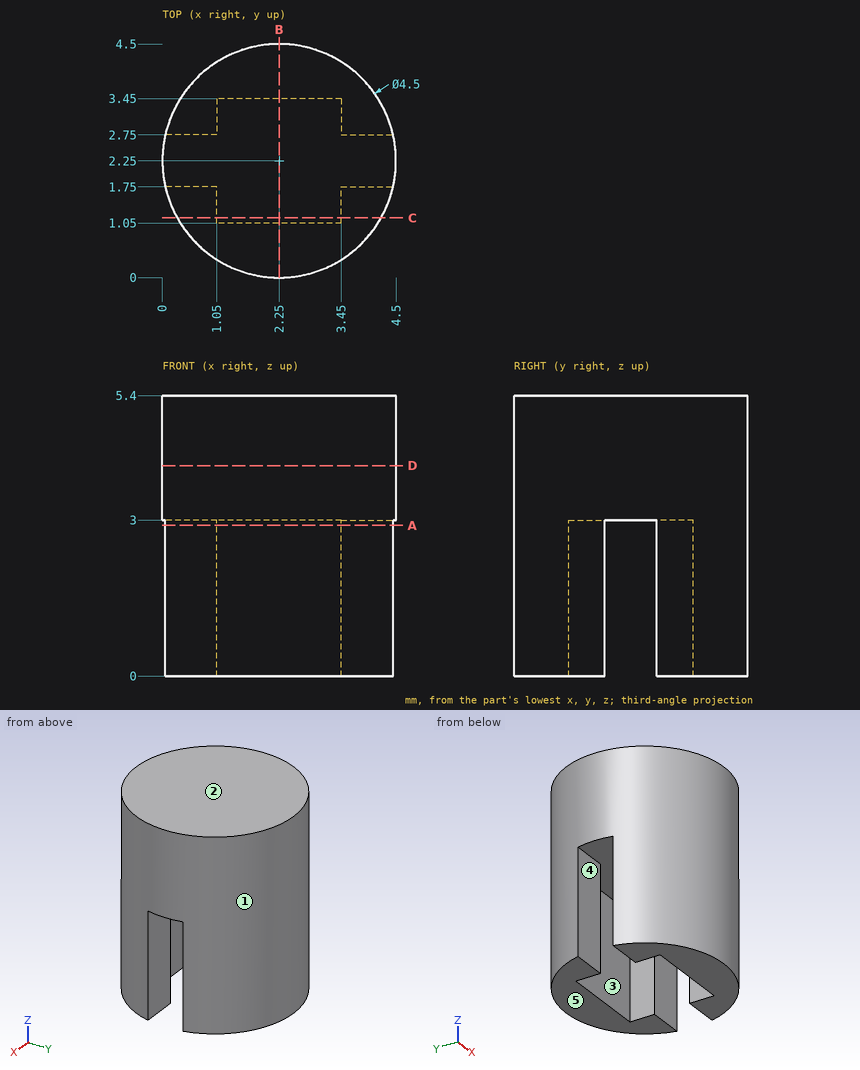
Print and shaded views of the part. All mm, measured from the part's lowest x, y and z. A direction names the side the tool comes from. Give positions to 0.01 mm unless a question says otherwise; leave off trailing zeros. Loops run counter-clockwise (first coordinate to the right, second up) from the corner with the lowest first, then second, coordinate; pieces in that order, holes last. Notation, with made-up numbers: M -28.5,-36 L 20.5,-36 A20 ccw 20.5,-31 Z; hole C 56.5,-4 d2. An arc over 180 degrees is marked long. Write each question's results on one line, items separated by ' | '.
Q1. Probe probe 1 along Y at (x, z) = (2.3, 2.35); probe 2 along Y at (x, z) = (0.8, 2.6); probe 3 along Z at (x, y) = (1.15, 3.35). List the from-to ranges inside material, lowest first.
Geometry check:
probe 1: y = 0 to 1.05, 3.45 to 4.5 | probe 2: y = 0.53 to 1.75, 2.75 to 3.97 | probe 3: z = 3 to 5.4
Q2. Flat gauge pins, fed straight in: P1, Ø1.9, axis at x = 2.5, z = 2, coming from the -Y side; P2, Ø0.5, axis at x = 0.5, z = 1.5, coming from the -Y side; P3, Ø0.5, axis at x = 4, z = 1, coming from the +Y side; P4, Ø0.8, axis at x = 0.5, z = 2, coming from the +Y side. Where does each tip first touch, or does it go through?
Geometry check:
P1: stops at y = 0 | P2: stops at y = 0.57 | P3: stops at y = 3.93 | P4: stops at y = 4.05
Q3. Band-saw the part on B-B on x = 2.25. Write the cut outline in (y, z).
Geometry check:
outline: M 0,0 L 1.05,0 L 1.05,3 L 3.45,3 L 3.45,0 L 4.5,0 L 4.5,5.4 L 0,5.4 Z
Q4. Band-saw the part on D-D on z = 4.05. Write the cut outline in (x, y).
Geometry check:
outline: C 2.25,2.25 d4.5
Q5. Which spindle directions (+Z, -Z, +X, -X, +Y, -Y) get a long thin tool onto all of the face, cutting with end or side? Do the marked faces 4 and 5. Say none if no direction does.
Geometry check:
face 4: -Z, +X, -X | face 5: -Z, +X, -X, +Y, -Y
Q6. Mould opens along X. For the marked faces 1, 2 and 3 say: pulls with the +X half, pulls with the -X half, needs draft (parallel to the pull), parting line crosses it, or undercut.
Geometry check:
face 1: parting line crosses it | face 2: needs draft | face 3: undercut
Q7. Band-saw the part on C-C on y = 1.15. Write the cut outline in (x, z).
Geometry check:
outline: M 0.29,0 L 1.05,0 L 1.05,3 L 3.45,3 L 3.45,0 L 4.21,0 L 4.21,5.4 L 0.29,5.4 Z
Q8. Band-saw the part on A-A on z = 2.9. Write the cut outline in (x, y).
Geometry check:
outline: M 0.06,1.75 A2.25 ccw 4.44,1.75 L 3.45,1.75 L 3.45,1.05 L 1.05,1.05 L 1.05,1.75 Z; M 0.06,2.75 L 1.05,2.75 L 1.05,3.45 L 3.45,3.45 L 3.45,2.75 L 4.44,2.75 A2.25 ccw Z
